Can you work these out from the model? Positions are in its coordinate system, mm. A direction names the side the tool comes from. Give positions to 0.01 mm unless a question says otherwise; leave off trailing zeros. Loops run counter-clockwise (first coordinate to the right, second up) from the corner with the lowest first, then second, coordinate; pieces in that order, holes last. Notation, with made-up numbers: M 81,28 L 91,28 A24 ccw 91,39 Z; hole C 74.25,32.5 d2. An arc over 180 degrees is marked long. One line per item, written item: value. Start each with the question number.
from build123d import *

# Parameters (mm, degrees)
F0_R     = 25.4
F0_R_2   = 12.7
F1_DEPTH = 76.2
F3_DEPTH = 27.94
F6_DEPTH = 12.7
F7_W     = 9.525
F7_H     = 10.5276096967
F7_H_2   = 16.1029547439
F8_DEPTH = 25.4


with BuildPart() as f1:
    # F0 (on Right) → F1 (new body)
    with BuildSketch(Plane.YZ):
        Circle(F0_R)
        Circle(F0_R_2, mode=Mode.SUBTRACT)
    extrude(amount=F1_DEPTH)

    # F2 (on Front) → F3 (cut, symmetric)
    with BuildSketch(Plane.XZ):
        Polygon((76.2, 25.4), (50.8, 25.4), (50.8, -9.525), (63.5, -9.525), (63.5, 9.525), (76.2, 9.525), align=None)
    extrude(amount=F3_DEPTH, both=True, mode=Mode.SUBTRACT)

    # F5 (on offset) → F6 (join)
    with BuildSketch(Plane.XZ.offset(-25.4)):
        Polygon((0, 0), (38.1, 0), (0, 50.8), align=None)
    extrude(amount=F6_DEPTH)

    # F7 (on face) → F8 (join)
    with BuildSketch(Plane.XZ.offset(-12.7)):
        with Locations((4.7625, 16.7332404078)):
            Rectangle(F7_W, F7_H)
        Polygon((21.6022160579, 21.9970452561), (9.525, 38.1), (9.525, 21.9970452561), align=None)
        with Locations((4.7625, 30.0485226281)):
            Rectangle(F7_W, F7_H_2)
    extrude(amount=F8_DEPTH)


solid = f1.part
Q1. For P1, Ø4, axis at x = 58, y = 15.5, coming from the +Z side (3 decimals); P2, Ø5, axis at x = 4, z = 47.5, coming from the -Y side; P3, Ø3, axis at x = 31.5, z = -4.5, coming from the +Y side, each with a flat end and sliding along its axis, tell me the tip position at first contact or that it passes through.
Q2. If we section it at B-B, the plane x = 15: Write out the boundary of the cut face in (y, z), plus the area to 3 significant figures.
Q3. I need wall thicknesses on line 1 along X through (y, z) = (-20, 3); line 2 along Z through (x, y) = (29, 0). Which ranges of each line are inside material? Lowest first, please.
Q4. If we mould it in two halves opening along X, with no side actions, what happens to faces 6 (the face through (76.2, 5, -12)), 7 (the face through (10, 25.4, 14)), 8 (the face through (63.5, 19, 0))? For each: released by +X, released by -X, zero draft, split by the parting line, or undercut.
Q5. If we section it at C-C, the plane y = -14: Write out the boundary of the cut face in (x, z) (3 decimals), plus the area to 3 significant figures.
Q6. If we section it at D-D, the plane z = 20.5: Write out the boundary of the cut face in (x, y) (3 decimals).
Q7. Which directions (+Z, -Z, +X, -X, +Y, -Y) give clear straight access to the entire face, cutting with the end or side of a thin tool? Please do faces 1 (the face through (50.8, 5, 12)), 2 (the face through (0, 5, 13)), 3 (the face through (70, -16, 9.525)), 4 (the face through (8, -12.7, 28)), 5 (the face through (5, 0, 11.469)).
Q8. If we section it at A-A, the plane y = 0: Write out the boundary of the cut face in (x, z) (3 decimals).
Response:
1. P1: z = -9.525
1. P2: y = 12.7
1. P3: y = 25.22
2. outline: M -12.7,22 A25.4 ccw long 25.4,0 L 25.4,30.8 L -12.7,30.8 Z; hole C 0,0 d25.4
2. area: 1,880 mm^2
3. line 1: 0 to 50.8, 63.5 to 76.2
3. line 2: -25.4 to -12.7, 12.7 to 25.4
4. face 6: released by +X
4. face 7: zero draft
4. face 8: undercut
5. outline: M 0,-21.193 L 76.2,-21.193 L 76.2,9.525 L 63.5,9.525 L 63.5,-9.525 L 50.8,-9.525 L 50.8,21.193 L 0,21.193 Z
5. area: 2,690 mm^2
6. outline: M 0,-14.997 L 50.8,-14.997 L 50.8,14.997 L 22.725,14.997 L 22.725,25.4 L 0,25.4 Z
7. face 1: +Z, +Y, -Y
7. face 2: +Z, -Z, -X, +Y, -Y
7. face 3: +Z, +X, +Y, -Y
7. face 4: +Z, +X, -X, -Y
7. face 5: +X, -X
8. outline: M 0,-25.4 L 76.2,-25.4 L 76.2,-12.7 L 0,-12.7 Z; M 0,11.469 L 9.525,11.469 L 9.525,12.7 L 50.8,12.7 L 50.8,25.4 L 19.05,25.4 L 9.525,38.1 L 0,38.1 Z
